For this review, take the finished solid that the model builds, in its own axes (mm). Face numbers are marked on the shaded views. A direction names the side the tool comes from. Give positions to 0.01 mm unless a question says otherwise; leave off trailing zeros. Write each loop counter-clockwise with the first axis right and the second up, starting at its lowest first coordinate (ties: lowest second). Pieces come first, ordered by that corner, then holes.
1) We need section A-A on x = 0. Give the boundary of the cut face in (y, z), and give its area (3 significant figures).
2) Machinability: for the marked faces 5 and 6, which of the approach directions +Z, -Z, +X, -X, +Y, -Y give a long, thin tool a straight path to every point of the face, cutting with its end or side? Answer none if there is none.
3) Draft analysis for pull direction X (two halves, no side actions). For the marked faces 1, 2, 3 and 4, state which applies: pulls with the +X half, pulls with the -X half, needs draft (parallel to the pull), parting line crosses it, or undercut.
4) We need section C-C on z = 0.7. Give the boundary of the cut face in (x, y).
5) Wall thickness on line 1 along Z through (x, y) = (-2.5, 1.5); line 2 along Y through (x, z) = (-0.25, 1.15); line 3 along Y through (x, z) = (0.5, 1.3): over which ranges is each line inside the solid? List them lowest first.
6) For P1, Ø1, axis at y = -3, z = 0, coming from the +X side, flat-tipped, find the tip position at first contact; note if it passes through.
7) We need section B-B on y = 0. Give the boundary of the cut face in (x, z).
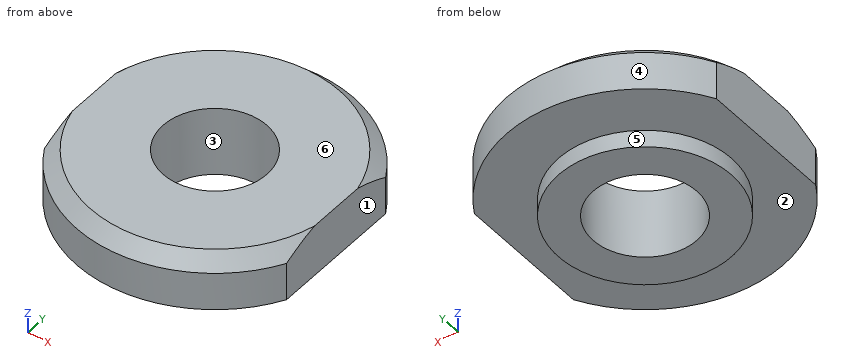
from build123d import *

# Parameters (mm, degrees)
BOSS_EXTRUDE1_DEPTH   = 1.5
SKETCH3_R             = 2.5
BOSS_EXTRUDE2_DEPTH   = 0.5
CHAMFER1_SIZE         = 0.4
F_3_0MM_DOWEL_HOLE1_D = 3


with BuildPart() as part:
    # Sketch1 → Boss-Extrude1 (new body)
    with BuildSketch(Plane.XY):
        with BuildLine():
            Line((-3.5, 1.936491673), (-3.5, -1.936491673))
            ThreePointArc((-3.5, -1.936491673), (0, -4), (3.5, -1.936491673))
            Line((3.5, -1.936491673), (3.5, 1.936491673))
            ThreePointArc((3.5, 1.936491673), (0, 4), (-3.5, 1.936491673))
        make_face()
    extrude(amount=BOSS_EXTRUDE1_DEPTH)

    # Sketch3 → Boss-Extrude2 (add)
    with BuildSketch(Plane(origin=(0, 0, 0), x_dir=(-1, 0, 0), z_dir=(0, 0, -1))):
        Circle(SKETCH3_R)
    extrude(amount=BOSS_EXTRUDE2_DEPTH)

    # Chamfer1
    chamfer1_edges = [part.edges().sort_by_distance(p)[0] for p in [
        (0, 4, 1.5),
        (0, -4, 1.5),
    ]]
    chamfer(chamfer1_edges, length=CHAMFER1_SIZE)

    # Ø3.0mm Dowel Hole1 (through all)
    with Locations(Plane.XY.offset(1.5)):
        with Locations((0, 0)):
            Hole(F_3_0MM_DOWEL_HOLE1_D / 2)


solid = part.part
Results list:
1. outline: (-4, 0) - (-2.5, 0) - (-2.5, -0.5) - (-1.5, -0.5) - (-1.5, 1.5) - (-3.6, 1.5) - (-4, 1.1) - close; (1.5, -0.5) - (2.5, -0.5) - (2.5, 0) - (4, 0) - (4, 1.1) - (3.6, 1.5) - (1.5, 1.5) - close
1. area: 8.34 mm2
2. face 5: -Z
2. face 6: +Z, +X, -X, +Y, -Y
3. face 1: pulls with the +X half
3. face 2: needs draft
3. face 3: undercut
3. face 4: parting line crosses it
4. outline: (-3.5, -1.94) arc R4 ccw to (3.5, -1.94) - (3.5, 1.94) arc R4 ccw to (-3.5, 1.94) - close; hole circle Ø3 at (0, 0)
5. line 1: z = 0 to 1.5
5. line 2: y = -3.94 to -1.48, 1.48 to 3.94
5. line 3: y = -3.77 to -1.41, 1.41 to 3.77
6. P1: stops at x = 3.12
7. outline: (-3.5, 0) - (-2.5, 0) - (-2.5, -0.5) - (-1.5, -0.5) - (-1.5, 1.5) - (-3.5, 1.5) - close; (1.5, -0.5) - (2.5, -0.5) - (2.5, 0) - (3.5, 0) - (3.5, 1.5) - (1.5, 1.5) - close
